```python
from build123d import *

# Parameters (mm, degrees)
SKETCH2_R          = 12.319
CUT_EXTRUDE2_DEPTH = 15.5448
SKETCH3_R          = 10.9855
CUT_EXTRUDE3_DEPTH = 40.253479183


with BuildPart() as part:
    # Sketch1 → Revolve2 (revolve)
    with BuildSketch(Plane.XY):
        Polygon((-18.542, 15.5448), (-17.526, 15.5448), (-17.526, 0), (0, 0), (0, 29.21), (-12.6365, 29.21), (-12.6365, 25.0698), (-18.542, 25.0698), align=None)
    revolve(axis=Axis((0, 29.21, 0), (0, -1, 0)))

    # Sketch2 → Cut-Extrude2 (cut)
    with BuildSketch(Plane.XZ):
        with Locations(Location((0, 0, 0), (0, 0, 270))):
            Circle(SKETCH2_R)
    extrude(amount=-CUT_EXTRUDE2_DEPTH, mode=Mode.SUBTRACT)

    # Sketch3 → Cut-Extrude3 (cut, through all)
    with BuildSketch(Plane(origin=(0, 29.21, 0), x_dir=(1, 0, 0), z_dir=(0, 1, 0))):
        with Locations(Location((0, 0, 0), (0, 0, 270))):
            Circle(SKETCH3_R)
    extrude(amount=-CUT_EXTRUDE3_DEPTH, mode=Mode.SUBTRACT)


solid = part.part
```
Model file for the job. Use its own axes, mm. A direction names the side the tool comes from. Coordinates: 2 decimals unless noted, no trailing zeros. Order: outer loops, then holes, each group sorted by start corner. A loop starts at its lowest first (then second) coordinate and runs counter-clockwise, first axis right, second up. Notation, with made-up numbers: (64, -7.5) -> (90, -7.5) arc R25 ccw to (90, 29.5) -> close; hole circle Ø9 at (74, -8). An arc over 180 degrees is marked (long way). Return JSON: item names as keys, results as strings.
Item 1: Slice it at C-C (y = 10.75). Write the cut outline in (x, z).
Model answer:
{"outline": "circle Ø35.05 at (0, 0); hole circle Ø24.64 at (0, 0)"}
Item 2: Slice it at B-B (z = 3). Write the cut outline in (x, y).
Model answer:
{"outline": "(-18.3, 15.54) -> (-17.27, 15.54) -> (-17.27, 0) -> (-11.95, 0) -> (-11.95, 15.54) -> (-10.57, 15.54) -> (-10.57, 29.21) -> (-12.28, 29.21) -> (-12.28, 25.07) -> (-18.3, 25.07) -> close; (10.57, 15.54) -> (11.95, 15.54) -> (11.95, 0) -> (17.27, 0) -> (17.27, 15.54) -> (18.3, 15.54) -> (18.3, 25.07) -> (12.28, 25.07) -> (12.28, 29.21) -> (10.57, 29.21) -> close"}
Item 3: Wall check: line 1 along X through (y, z) = (19.5, 0); line 2 along X through (y, z) = (2.25, -0.5); line 3 along Y through (x, z) = (12, 2.5). Give the ranges that are in metal, low to high. Write a range as from..to.
Model answer:
{"line 1": "x = -18.54..-10.99, 10.99..18.54", "line 2": "x = -17.52..-12.31, 12.31..17.52", "line 3": "y = 15.54..29.21"}
Item 4: Slice it at A-A (x = 0). Write the cut outline in (y, z).
Model answer:
{"outline": "(0, -17.53) -> (15.54, -17.53) -> (15.54, -18.54) -> (25.07, -18.54) -> (25.07, -12.64) -> (29.21, -12.64) -> (29.21, -10.99) -> (15.54, -10.99) -> (15.54, -12.32) -> (0, -12.32) -> close; (0, 12.32) -> (15.54, 12.32) -> (15.54, 10.99) -> (29.21, 10.99) -> (29.21, 12.64) -> (25.07, 12.64) -> (25.07, 18.54) -> (15.54, 18.54) -> (15.54, 17.53) -> (0, 17.53) -> close"}
Item 5: Mould opens along X. For faces 1 (the face through (-10.93, 7.66, -5.68)), 2 (the face through (-4.4, 25.07, 12.1)), 3 (the face through (-16.72, 7.66, -5.26)) say: pulls with the +X half, pulls with the -X half, needs draft (parallel to the pull), parting line crosses it, or undercut.
Model answer:
{"face 1": "undercut", "face 2": "needs draft", "face 3": "parting line crosses it"}
Item 6: Pin check, flat tips, straight feed: P1, Ø10, axis at x = 13.5, y = 3.5, coming from the +Z side; P2, Ø6, axis at x = -2.5, y = 9, coming from the +Z side; P3, Ø5, axis at y = 7, z = 8.5, coming from the -X side; P4, Ø17.5, axis at x = 0, z = 0, coming from the -Y side. Stop position of each tip, or through.
Model answer:
{"P1": "stops at z = 15.33", "P2": "stops at z = 17.53", "P3": "stops at x = -16.47", "P4": "passes through"}
Item 7: Slice it at D-D (x = -16). Write the cut outline in (y, z).
Model answer:
{"outline": "(0, -7.15) -> (15.54, -7.15) -> (15.54, -9.37) -> (25.07, -9.37) -> (25.07, 9.37) -> (15.54, 9.37) -> (15.54, 7.15) -> (0, 7.15) -> close"}
Item 8: 3-axis set-ups, long thin cutter, end or side, ignore diameter. For faces 4 (the face through (3.3, 22.47, 10.48)), 5 (the face through (-5.83, 27.11, 11.21)), 6 (the face through (-2, 15.545, 11)): which of +Z, -Z, +X, -X, +Y, -Y reach the whole face in a straight line?
Model answer:
{"face 4": "+Y, -Y", "face 5": "+Y", "face 6": "-Y"}
